Input: part model. Units: mm. Frame: model coordinates. A direction names the side the tool comes from. Coordinates: 2 decimals unless noted, no trailing zeros. Write each loop counter-clockwise with the first axis right and the second up, starting at its lowest first coordinate (ties: lowest second). Pieces come first, ordered by that corner, then holes. Notation, with made-up numbers: M 37,57 L 53,57 A18 cw 53,84 Z; hole C -8,-12.5 d6. An arc over 180 degrees is marked long. Write each question's results on one line, items separated by ' | '. Start each with the question number.
1. Section query B-B, the plane y = 14. Output: boundary loops of the cut face in (x, z), and give its area (4 significant figures).
2. Section query D-D, the plane y = -0.25. Output: boundary loops of the cut face in (x, z).
3. Pull-direction query (X, two-part tool) for faces 1 (the flat face through (-23.824, 9, 2)), 2 (the flat face through (-6.971, 18.9, 3.6)), 3 (the flat face through (-11, 10, 0)); classes: +X half, -X half, draft (parallel to the pull), parting line (faces both ways), or undercut.
4. Set-up query: faces 4 (the flat face through (-4, 19, 3.1)), 5 (the flat face through (-16.324, 10, 7)), 6 (the flat face through (-6.324, 10, 7)). Return all of +Z, -Z, +X, -X, +Y, -Y with unobstructed straight access to the full face (end or side cutting, diameter ignored); none if empty.
5. Ray query, probe 1 along Y at (x, z) = (-5.25, 4); probe 2 along Z at (x, y) = (-11.75, 16.5); probe 3 along Z at (x, y) = (-2.75, 19.5). Return the intervals inside material, ascending.
6. Section query C-C, the plane z = 6. Output: boundary loops of the cut face in (x, y).
7. First-contact query: pin 1 (5.5 mm diameter, centred on x = -11, z = 7, fed in from -Y); pin 2 (1.5 mm diameter, centred on x = -5, y = 13, fed in from +Z); pin 3 (3.5 mm diameter, centred on x = -11, z = 6.5, fed in from +Y). Flat tips, straight axial feed; report the tip coordinate or a pass-through.
8. Section query A-A, the plane x = -5. Output: boundary loops of the cut face in (y, z), and give its area (3 significant figures).
```python
from build123d import *

# Parameters (mm, degrees)
SKETCH_1_W          = 25
SKETCH_1_H          = 25
EXTRUDE_1_DEPTH     = 4.1
SKETCH_2_W          = 10
SKETCH_2_H          = 10
EXTRUDE_2_DEPTH     = 6.6
SKETCH_3_W          = 5.758400008
SKETCH_3_H          = 3.721892688
CUT_EXTRUDE_1_DEPTH = 1


with BuildPart() as part:
    # 草图1 → 凸台-拉伸1 (new body)
    with BuildSketch(Plane.XY):
        with Locations((-11.324496329, 9.624744468)):
            Rectangle(SKETCH_1_W, SKETCH_1_H)
    extrude(amount=EXTRUDE_1_DEPTH)

    # 草图2 → 凸台-拉伸2 (add)
    with BuildSketch(Plane.XY.offset(4.1)):
        with Locations((-11.324496329, 10.424744468)):
            Rectangle(SKETCH_2_W, SKETCH_2_H)
    extrude(amount=EXTRUDE_2_DEPTH)

    # 草图3 → 切除-拉伸1 (cut)
    with BuildSketch(Plane.XY.offset(4.1)):
        with Locations((-4.091384125, 18.91192009)):
            Rectangle(SKETCH_3_W, SKETCH_3_H)
    extrude(amount=-CUT_EXTRUDE_1_DEPTH, mode=Mode.SUBTRACT)


solid = part.part
```
Answer:
1) outline: M -23.82,0 L 1.18,0 L 1.18,4.1 L -6.32,4.1 L -6.32,10.7 L -16.32,10.7 L -16.32,4.1 L -23.82,4.1 Z | area: 168.5 mm^2
2) outline: M -23.82,0 L 1.18,0 L 1.18,4.1 L -23.82,4.1 Z
3) face 1: -X half | face 2: undercut | face 3: draft
4) face 4: +Z | face 5: +Z, -X, +Y, -Y | face 6: +Z, +X, +Y, -Y
5) probe 1: -2.88 to 17.05, 20.77 to 22.12 | probe 2: 0 to 4.1 | probe 3: 0 to 3.1
6) outline: M -16.32,5.42 L -6.32,5.42 L -6.32,15.42 L -16.32,15.42 Z
7) pin 1: y = 5.42 | pin 2: z = 4.1 | pin 3: y = 15.42
8) outline: M -2.88,0 L 22.12,0 L 22.12,4.1 L 20.77,4.1 L 20.77,3.1 L 17.05,3.1 L 17.05,4.1 L -2.88,4.1 Z | area: 98.8 mm^2
